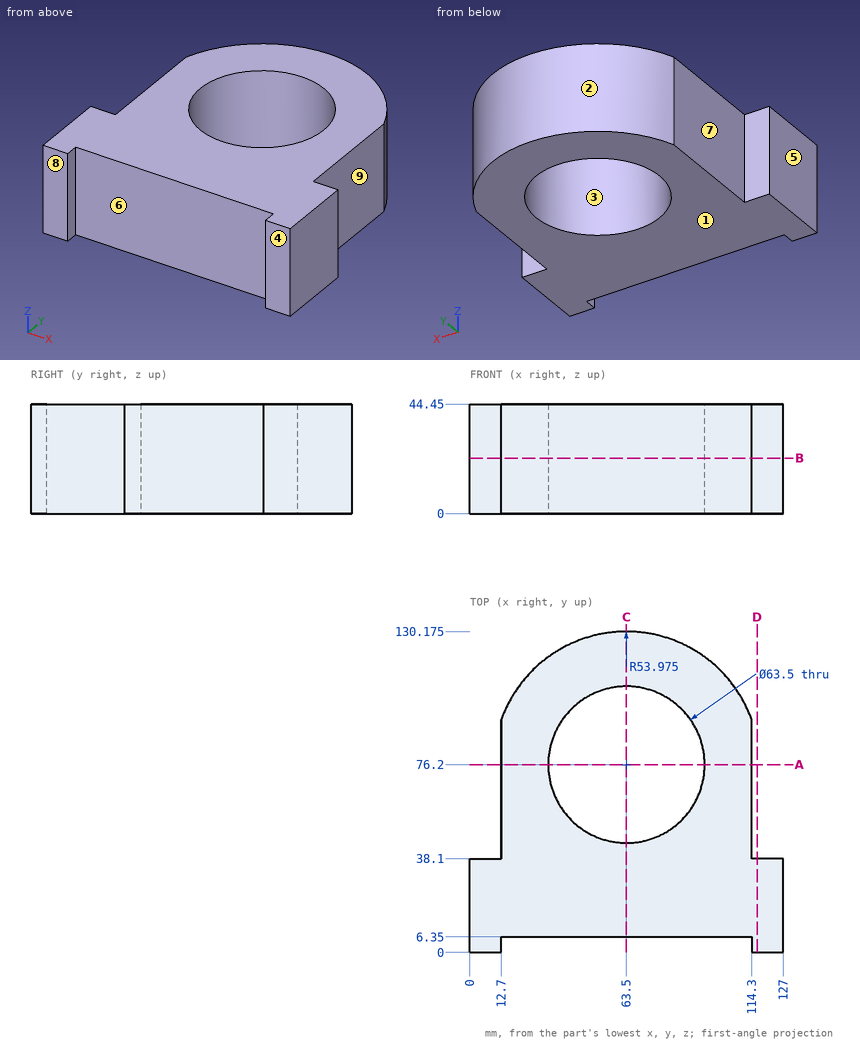
For this review, use the dimensioned drawing (mm, ordinates from the lowest corner) and the shaded views. A direction names the side the tool comes from. Coordinates: 2 decimals unless noted, no trailing zeros. Loops run counter-clockwise (first coordinate to the right, second up) from the corner with the lowest first, then second, coordinate; pieces in that order, holes last. Notation, with made-up numbers: (-23, 69.25) -> (-7, 69.25) arc R18 cw to (-7, 78.25) -> close; hole circle Ø1 at (-39.5, 68). An arc over 180 degrees is marked (long way). Use a Markdown table: item, result. Add a question column.
Item 1: Wall thickness on L1, parallel to Y at x = 63.5, z = 11 (3 decimals); L2, parallel to X at y = 76, z = 9; L3, parallel to X at y = 59, z = 30: over which ranges is each line inside the solid? List them lowest first. Write a range as from..to.
Item 2: We need section D-D, the plane x = 116.5. Write out the cut boundary in (y, z).
Item 3: We need section B-B, the plane z = 22.5. Write out the cut boundary in (x, y) (3 decimals), and give its area (3 significant figures).
Item 4: Clearance check with flat-ended pins moving along their axes: P1, Ø10, axis at x = 8.5, z = 13, coming from the +Y side; P2, Ø6, axis at x = 83, z = 31, coming from the -Y side; P3, Ø5, axis at y = 57.5, z = 39.5, coming from the +X side. State where each tip first meets the part, or that it passes through.
Item 5: Machinability: for the marked faces 5, 6, 7, 8 and 9, which of the approach directions +Z, -Z, +X, -X, +Y, -Y give a long, thin tool a straight path to every point of the face, cutting with its end or side? Answer none if there is none.
Item 6: We need section A-A, the plane y = 76.2. Write out the cut boundary in (x, z).
Item 7: The part is to be moulded in two halves that separate along Y. For the marked faces 1, 2, 3 and 4, say which applies: +Y half, -Y half, draft (parallel to the pull), parting line (faces both ways), or undercut.
Item 8: We need section C-C, the plane x = 63.5. Write out the cut boundary in (y, z) (3 decimals), and give its area (3 significant figures).
Numbers:
| question | item | result |
|---|---|---|
| 1 | L1 | y = 6.35..44.45, 107.95..130.175 |
| 1 | L2 | x = 12.7..31.75, 95.25..114.3 |
| 1 | L3 | x = 12.7..36.81, 90.19..114.3 |
| 2 | outline | (0, 0) -> (38.1, 0) -> (38.1, 44.45) -> (0, 44.45) -> close |
| 3 | outline | (0, 0) -> (12.7, 0) -> (12.7, 6.35) -> (114.3, 6.35) -> (114.3, 0) -> (127, 0) -> (127, 38.1) -> (114.3, 38.1) -> (114.3, 94.439) arc R53.975 ccw to (12.7, 94.439) -> (12.7, 38.1) -> (0, 38.1) -> close; hole circle Ø63.5 at (63.5, 76.2) |
| 3 | area | 9,400 mm^2 |
| 4 | P1 | stops at y = 96.53 |
| 4 | P2 | stops at y = 6.35 |
| 4 | P3 | stops at x = 114.3 |
| 5 | face 5 | +Z, -Z, -X, +Y, -Y |
| 5 | face 6 | +Z, -Z, -Y |
| 5 | face 7 | +Z, -Z, -X, +Y |
| 5 | face 8 | +Z, -Z, +X, -X, -Y |
| 5 | face 9 | +Z, -Z, +X, +Y |
| 6 | outline | (12.7, 0) -> (31.75, 0) -> (31.75, 44.45) -> (12.7, 44.45) -> close; (95.25, 0) -> (114.3, 0) -> (114.3, 44.45) -> (95.25, 44.45) -> close |
| 7 | face 1 | draft |
| 7 | face 2 | +Y half |
| 7 | face 3 | undercut |
| 7 | face 4 | -Y half |
| 8 | outline | (6.35, 0) -> (44.45, 0) -> (44.45, 44.45) -> (6.35, 44.45) -> close; (107.95, 0) -> (130.175, 0) -> (130.175, 44.45) -> (107.95, 44.45) -> close |
| 8 | area | 2,680 mm^2 |
